Could you check a few things on this model? Use its own coordinates, in mm. A direction names the side the tool comes from. Round coordinates to 2 decimals unless told otherwise and drop trailing zeros. Order: outer loops, then holes, each group sorted by start corner. A loop starts at its lowest first (then second) coordinate and runs counter-clockwise, first axis right, second up. Notation, with made-up numbers: (79, 17) - (122, 17) arc R31 ccw to (122, 50) - close; hole circle Ø3 at (5, -34.75). An arc over 180 degrees is marked (long way). Use one line per item in the form item = value.
from build123d import *

# Parameters (mm, degrees)
SKETCH1_W           = 139
SKETCH1_H           = 43
SKETCH1_R           = 3.1
SKETCH1_R_2         = 3.75
SKETCH1_R_3         = 1.6
SKETCH1_R_4         = 5.1
SKETCH1_W_2         = 2.7
SKETCH1_H_2         = 1.2
SKETCH1_W_3         = 2.2
SKETCH1_H_3         = 1.1
BOSS_EXTRUDE1_DEPTH = 3


with BuildPart() as part:
    # Sketch1 → Boss-Extrude1 (new body)
    with BuildSketch(Plane.XY):
        with Locations((69.5, 21.5)):
            Rectangle(SKETCH1_W, SKETCH1_H)
        with Locations((32.375644347, 31)):
            Circle(SKETCH1_R, mode=Mode.SUBTRACT)
        with Locations((94.5, 10)):
            Circle(SKETCH1_R_2, mode=Mode.SUBTRACT)
        with Locations((4, 32.5)):
            Circle(SKETCH1_R_3, mode=Mode.SUBTRACT)
        with Locations((135, 32.5)):
            Circle(SKETCH1_R_3, mode=Mode.SUBTRACT)
        with Locations((135, 10.5)):
            Circle(SKETCH1_R_3, mode=Mode.SUBTRACT)
        with Locations((4, 10.5)):
            Circle(SKETCH1_R_3, mode=Mode.SUBTRACT)
        with Locations((69.5, 21.5)):
            Circle(SKETCH1_R_4, mode=Mode.SUBTRACT)
        with Locations((15, 21.5)):
            Circle(SKETCH1_R_3, mode=Mode.SUBTRACT)
        with Locations((124, 21.5)):
            Circle(SKETCH1_R_3, mode=Mode.SUBTRACT)
        with Locations(Location((44.5, 10, 0), (0, 0, 180))):
            Circle(SKETCH1_R_2, mode=Mode.SUBTRACT)
        with Locations((106.624355653, 31)):
            Circle(SKETCH1_R_2, mode=Mode.SUBTRACT)
        with Locations((32.375644347, 25)):
            Rectangle(SKETCH1_W_2, SKETCH1_H_2, mode=Mode.SUBTRACT)
        with Locations((94.5, 3.75)):
            Rectangle(SKETCH1_W_3, SKETCH1_H_3, mode=Mode.SUBTRACT)
        with Locations((44.5, 3.75)):
            Rectangle(SKETCH1_W_3, SKETCH1_H_3, mode=Mode.SUBTRACT)
        with Locations((106.624355653, 24.75)):
            Rectangle(SKETCH1_W_3, SKETCH1_H_3, mode=Mode.SUBTRACT)
    extrude(amount=BOSS_EXTRUDE1_DEPTH)


solid = part.part
Item 1: If we mould it in two halves opening along X, with no side actions, what happens to faces 3 (the face through (107, 25.3, 1)), 4 (the face through (69, 27, 3)), 5 (the face through (0, 21, 1))? For each: released by +X, released by -X, zero draft, split by the parting line, or undercut.
Found:
face_3 = undercut
face_4 = zero draft
face_5 = released by -X
Item 2: Imagine slicing it at B-B on y = 21.5. Please give me the cut outline in (x, z), plus the area to 3 significant figures.
Found:
outline = (0, 0) - (13.4, 0) - (13.4, 3) - (0, 3) - close; (16.6, 0) - (64.4, 0) - (64.4, 3) - (16.6, 3) - close; (74.6, 0) - (122.4, 0) - (122.4, 3) - (74.6, 3) - close; (125.6, 0) - (139, 0) - (139, 3) - (125.6, 3) - close
area = 367 mm2
Item 3: For faces 1 (the face through (139, 21, 1)), 2 (the face through (32, 25.6, 1)), which set-ups out of +Z, -Z, +X, -X, +Y, -Y let a thin tool reach every point of the face, with its end or its side?
Found:
face_1 = +Z, -Z, +X, +Y, -Y
face_2 = +Z, -Z
Item 4: Imagine slicing it at A-A on x = 69.5. Please give me the cut outline in (y, z), plus the area to 3 significant figures.
Found:
outline = (0, 0) - (16.4, 0) - (16.4, 3) - (0, 3) - close; (26.6, 0) - (43, 0) - (43, 3) - (26.6, 3) - close
area = 98.4 mm2
Item 5: Imagine slicing it at C-C on x = 135. Please give me the cut outline in (y, z).
Found:
outline = (0, 0) - (8.9, 0) - (8.9, 3) - (0, 3) - close; (12.1, 0) - (30.9, 0) - (30.9, 3) - (12.1, 3) - close; (34.1, 0) - (43, 0) - (43, 3) - (34.1, 3) - close
Item 6: Will this pin go through, and if not, where does the flat tip stop? P1, Ø8, axis at x = 69.5, y = 21.5, coming from the +Z side.
Found:
P1 = through
Item 7: I need wall thicknesses on L1, parallel to Y at x = 4, z = 1.5; L2, parallel to X at y = 8, z = 1.9; L3, parallel to Y at x = 69.5, z = 2.15. Which ranges of each line are inside material? Lowest first, please.
Found:
L1 = 0 to 8.9, 12.1 to 30.9, 34.1 to 43
L2 = 0 to 41.33, 47.67 to 91.33, 97.67 to 139
L3 = 0 to 16.4, 26.6 to 43
Item 8: Imagine slicing it at D-D on z = 2.25. State how many separate pieces and enclosed holes the cut face has, plus the area to 3 significant figures.
Found:
separate_pieces = 1
enclosed_holes = 15
area = 5,670 mm2
